Geometry: final body of the model. Coordinates: model frame, mm. A direction names the side the tool comes from. Coordinates: 2 decimals unless noted, no trailing zeros. Write each loop counter-clockwise with the first axis right and the second up, starting at its lowest first coordinate (ties: lowest second). Pieces come first, ordered by that corner, then holes. Notation, with made-up numbers: (-39, 57.25) - (-14, 57.25) arc R10 ccw to (-14, 73.25) - close; hole circle Ø4 at (-36.75, 49.25). An arc over 180 degrees is marked (long way). Answer as a JSON object with one key per item and string values. Group by question number.
Item 1: Section A-A on x = 45. Return loops of the section in (y, z) (3 decimals), and give its area (3 significant figures).
Item 2: First-contact query: pin 1 Ø1 at (x, z) = (-33, 24.5) entering from -Y; pin 2 Ø3 at (y, z) = (2.5, -21) entering from -X (3 decimals); pin 3 Ø1.9 at (y, z) = (2, -25.5) entering from +X (3 decimals). Flat tips, straight axial feed; report the tip coordinate or a pass-through.
Item 3: Line query: line 1 along X through (y, z) = (1, 29) (3 decimals); line 2 along Z through (x, y) = (96, 6) (3 decimals); line 3 along Z through (x, y) = (90, 4.5) (3 decimals). Output: solid intervals per line, ascending. Write a range as from..to.
Item 4: Set-up query: faces 4 (the flat face through (-121, 3, 6.35)), 5 (the flat face through (20, 3, 23.953)), 6 (the flat face through (66.675, 3, 32)). Return all of +Z, -Z, +X, -X, +Y, -Y with unobstructed straight access to the full face (end or side cutting, diameter ignored); none if empty.
Item 5: Mould query, pull axis Z, two halves, no side actions, for faces 1 (the flat face through (76, 3, 28.575)), 2 (the cylindrical face through (40.74, 3.22, 0.4)), 3 (the flat face through (-104.775, 3, 32)). Classes: pulls with the +Z half, pulls with the -Z half, needs draft (parallel to the pull), parting line crosses it, or undercut.
Item 6: Section B-B on z = -3. Return loops of the section in (x, y) (3 decimals), and give its area (3 significant figures).
Item 7: Section C-C on y = 2.5. State how many separate pieces and enclosed holes the cut face has, and give its area (3 significant figures).
```python
from build123d import *

# Parameters (mm, degrees)
ESQUISSE1_W                     = 234.95
ESQUISSE1_H                     = 57.15
BOSS_EXTRU_1_DEPTH              = 6.35
ENL_V_MAT_EXTRU_1_DEPTH         = 6.35
R_P_TITION_LIN_AIRE1_COUNT      = 6
R_P_TITION_LIN_AIRE1_PITCH      = 39.158333333
ESQUISSE3_W                     = 19.05
ESQUISSE3_H                     = 6.35
BOSS_EXTRU_2_DEPTH              = 6.35
R_P_TITION_LIN_AIRE2_COUNT      = 6
R_P_TITION_LIN_AIRE2_PITCH      = 38.1
ESQUISSE5_W                     = 6.35
ESQUISSE5_H                     = 12.7
BOSS_EXTRU_4_DEPTH              = 6.35
R_P_TITION_LIN_AIRE4_COUNT      = 2
R_P_TITION_LIN_AIRE4_PITCH      = 25.4
R_P_TITION_LIN_AIRE4_COUNT_DIR2 = 2
R_P_TITION_LIN_AIRE4_PITCH_DIR2 = 241.3


with BuildPart() as part:
    # Esquisse1 → Boss.-Extru.1 (new body)
    with BuildSketch(Plane(origin=(0, 0, 0), x_dir=(1, 0, 0), z_dir=(0, 1, 0))):
        Rectangle(ESQUISSE1_W, ESQUISSE1_H)
    extrude(amount=BOSS_EXTRU_1_DEPTH)

    # Esquisse2 → Enlèv. mat.-Extru.1 (cut)
    with BuildSketch(Plane(origin=(0, 6.35, 0), x_dir=(1, 0, 0), z_dir=(0, 1, 0))):
        with BuildLine():
            Line((93.704833333, 17.50529974), (93.704833333, 23.953124941))
            Line((93.704833333, 23.953124941), (102.086833333, 23.953124941))
            Line((102.086833333, 23.953124941), (102.086833333, 17.50529974))
            ThreePointArc((102.086833333, 17.50529974), (115.89571511, -0.065238332), (101.959833333, -17.535218961))
            Line((101.959833333, -17.535218961), (101.959833333, -23.953124941))
            Line((101.959833333, -23.953124941), (93.831833333, -23.953124941))
            Line((93.831833333, -23.953124941), (93.831833333, -17.535218961))
            ThreePointArc((93.831833333, -17.535218961), (79.895951557, -0.065238332), (93.704833333, 17.50529974))
        make_face()
    enl_v_mat_extru_1 = extrude(amount=-ENL_V_MAT_EXTRU_1_DEPTH, mode=Mode.SUBTRACT)

    # Répétition linéaire1: Enlèv. mat.-Extru.1 ×6
    with Locations(*[(-i * R_P_TITION_LIN_AIRE1_PITCH, 0, 0) for i in range(1, R_P_TITION_LIN_AIRE1_COUNT)]):
        add(enl_v_mat_extru_1, mode=Mode.SUBTRACT)

    # Esquisse3 → Boss.-Extru.2 (add)
    with BuildSketch(Plane(origin=(0, 6.35, 0), x_dir=(1, 0, 0), z_dir=(0, 1, 0))):
        with Locations((-95.25, -31.75)):
            Rectangle(ESQUISSE3_W, ESQUISSE3_H)
    boss_extru_2 = extrude(amount=-BOSS_EXTRU_2_DEPTH)

    # Répétition linéaire2: Boss.-Extru.2 ×6
    with Locations(*[(i * R_P_TITION_LIN_AIRE2_PITCH, 0, 0) for i in range(1, R_P_TITION_LIN_AIRE2_COUNT)]):
        add(boss_extru_2)

    # Esquisse5 → Boss.-Extru.4 (add)
    with BuildSketch(Plane(origin=(0, 6.35, 0), x_dir=(1, 0, 0), z_dir=(0, 1, 0))):
        with Locations((-120.65, -12.7)):
            Rectangle(ESQUISSE5_W, ESQUISSE5_H)
    boss_extru_4 = extrude(amount=-BOSS_EXTRU_4_DEPTH)

    # Répétition linéaire4: Boss.-Extru.4 2 × 2
    with Locations(*[(j * R_P_TITION_LIN_AIRE4_PITCH_DIR2, 0, -i * R_P_TITION_LIN_AIRE4_PITCH) for i in range(R_P_TITION_LIN_AIRE4_COUNT) for j in range(R_P_TITION_LIN_AIRE4_COUNT_DIR2) if (i, j) != (0, 0)]):
        add(boss_extru_4)


solid = part.part
```
Checks:
{
 "1": {"outline": "(0, -28.575) - (6.35, -28.575) - (6.35, -11.631) - (0, -11.631) - close; (0, 11.631) - (6.35, 11.631) - (6.35, 28.575) - (0, 28.575) - close", "area": "215 mm^2"},
 "2": {"pin 1": "y = 0", "pin 2": "x = -117.475", "pin 3": "x = 117.475"},
 "3": {"line 1": "-104.775..-85.725, -66.675..-47.625, -28.575..-9.525, 9.525..28.575, 47.625..66.675, 85.725..104.775", "line 2": "-28.575..-23.953, 23.953..34.925", "line 3": "-28.575..-16.176, 16.176..34.925"},
 "4": {"face 4": "-X, +Y, -Y", "face 5": "+Y, -Y", "face 6": "+Z, +Y, -Y"},
 "5": {"face 1": "pulls with the +Z half", "face 2": "undercut", "face 3": "needs draft"},
 "6": {"outline": "(-117.475, 0) - (-115.644, 0) - (-115.644, 6.35) - (-117.475, 6.35) - close; (-80.148, 0) - (-76.486, 0) - (-76.486, 6.35) - (-80.148, 6.35) - close; (-40.989, 0) - (-37.327, 0) - (-37.327, 6.35) - (-40.989, 6.35) - close; (-1.831, 0) - (1.831, 0) - (1.831, 6.35) - (-1.831, 6.35) - close; (37.327, 0) - (40.989, 0) - (40.989, 6.35) - (37.327, 6.35) - close; (76.486, 0) - (80.148, 0) - (80.148, 6.35) - (76.486, 6.35) - close; (115.644, 0) - (117.475, 0) - (117.475, 6.35) - (115.644, 6.35) - close", "area": "140 mm^2"},
 "7": {"separate pieces": "1", "enclosed holes": "6", "area": "7,760 mm^2"}
}
